Geometry check sheet. Reference: the model listing, model coordinates, mm. A direction names the side the tool comes from. Give positions to 0.01 mm unless a question says otherwise; leave off trailing zeros. Write each loop counter-clockwise with the first axis right and the second up, starting at its lowest first coordinate (ties: lowest second). Pieces come first, ordered by that corner, then holes. Notation, with made-up numbers: (-21.75, -16) - (34.25, -16) arc R25 ccw to (34.25, 18) - close; hole circle Ø4 at (32, 18.5). An arc over 180 degrees is marked (long way). One line per question, with ' | ' between items. Start each with the question number.
Q1. Set-up check for faces 1 (the face through (5.309, -99, 26)), 2 (the face through (71.725, -198.341, 2.691)), 3 (the face through (58, -183.388, 3)): record each of +Z, -Z, +X, -X, +Y, -Y from which the full face is reachable in a straight line by a thin tool's end or side.
Q2. Release check for a two-part mould opening along X. For faces 4 (the face through (58, -30.988, 3)), 5 (the face through (2.62, -1.81, 41.5)), 6 (the face through (0, -99, 23)) record: +X half, -X half, draft (parallel to the pull), parting line (faces both ways), or undercut.
Q3. Section check C-C on z = 32.5. Record the boundary of the cut face in (x, y).
Q4. Section check D-D on y = -179.5. Record the boundary of the cut face in (x, z).
Q5. Gauge pin test, flat ends, axial feed: P1, Ø19.5, axis at x = 45, y = -150, coming from the +Z side; P2, Ø5, axis at x = 35.5, z = 7, coming from the +Y side; P3, Ø13, axis at y = -74.68, z = 29.92, coming from the -X side. Record the tip position at first contact, or that the pin passes through.
Q6. Section check A-A on y = -73.5. Record the boundary of the cut face in (x, z), and give its area (3 significant figures).
Q7. Thickness scan on L1, parallel to Y at x = 53, z = 3.5; L2, parallel to Z at x = 22, y = -143.5. Record the ranges inside material, lowest first. Write a range as [from, to].
Q8. Section check B-B on y = -140. Record the boundary of the cut face in (x, z), and give its area (3 significant figures).
```python
from build123d import *

# Parameters (mm, degrees)
F1_DEPTH = 200.152
F3_D     = 14.3002
F4_R     = 6.35
F6_DEPTH = 25.4


with BuildPart() as f1:
    # F0 (on Front) → F1 (new body)
    with BuildSketch(Plane.XZ):
        with BuildLine():
            ThreePointArc((0, 2.794), (0.818344, 0.818344), (2.794, 0))
            Line((2.794, 0), (73.6346, 0))
            Line((73.6346, 0), (73.6346, 5.3086))
            Line((73.6346, 5.3086), (8.1026, 5.3086))
            ThreePointArc((8.1026, 5.3086), (6.126944, 6.126944), (5.3086, 8.1026))
            Line((5.3086, 8.1026), (5.3086, 43.4086))
            Line((5.3086, 43.4086), (0, 43.4086))
            Line((0, 43.4086), (0, 2.794))
        make_face()
    extrude(amount=F1_DEPTH)

    # F3 (through all)
    with Locations(Plane(origin=(0, 0, 0), x_dir=(0, -1, 0), z_dir=(-1, 0, 0))):
        with Locations((23.876, 29.9212), (74.676, 29.9212), (125.476, 29.9212), (176.276, 29.9212)):
            Hole(F3_D / 2)

    # F4
    f4_edges = [f1.edges().sort_by_distance(p)[0] for p in [
        (2.6543, 0, 43.4086),
        (73.6346, 0, 2.6543),
        (73.6346, -200.152, 2.6543),
        (2.6543, -200.152, 43.4086),
    ]]
    fillet(f4_edges, radius=F4_R)

    # F5 (on face) → F6 (cut)
    with BuildSketch(Plane.XY.offset(5.3086)):
        with BuildLine():
            ThreePointArc((66.3956, -23.876), (64.312543, -18.847057), (59.2836, -16.764))
            Line((59.2836, -16.764), (55.9816, -16.764))
            ThreePointArc((55.9816, -16.764), (50.952657, -18.847057), (48.8696, -23.876))
            ThreePointArc((48.8696, -23.876), (50.952657, -28.904943), (55.9816, -30.988))
            Line((55.9816, -30.988), (59.2836, -30.988))
            ThreePointArc((59.2836, -30.988), (64.312543, -28.904943), (66.3956, -23.876))
        make_face()
        with BuildLine():
            ThreePointArc((66.3956, -176.276), (64.312543, -171.247057), (59.2836, -169.164))
            Line((59.2836, -169.164), (55.9816, -169.164))
            ThreePointArc((55.9816, -169.164), (50.952657, -171.247057), (48.8696, -176.276))
            ThreePointArc((48.8696, -176.276), (50.952657, -181.304943), (55.9816, -183.388))
            Line((55.9816, -183.388), (59.2836, -183.388))
            ThreePointArc((59.2836, -183.388), (64.312543, -181.304943), (66.3956, -176.276))
        make_face()
    extrude(amount=-F6_DEPTH, mode=Mode.SUBTRACT)


solid = f1.part
```
Working result:
1) face 1: +Z, +X, +Y, -Y | face 2: +Z, -Z, +X, -Y | face 3: +Z, -Z
2) face 4: undercut | face 5: draft | face 6: -X half
3) outline: (0, -200.15) - (5.31, -200.15) - (5.31, -182.94) - (0, -182.94) - close; (0, -169.61) - (5.31, -169.61) - (5.31, -132.14) - (0, -132.14) - close; (0, -118.81) - (5.31, -118.81) - (5.31, -81.34) - (0, -81.34) - close; (0, -68.01) - (5.31, -68.01) - (5.31, -30.54) - (0, -30.54) - close; (0, -17.21) - (5.31, -17.21) - (5.31, 0) - (0, 0) - close
4) outline: (0, 2.79) arc R2.79 ccw to (2.79, 0) - (49.64, 0) - (49.64, 5.31) - (8.1, 5.31) arc R2.79 cw to (5.31, 8.1) - (5.31, 23.54) - (0, 23.54) - close; (0, 36.3) - (5.31, 36.3) - (5.31, 43.41) - (0, 43.41) - close; (65.62, 0) - (73.63, 0) - (73.63, 5.31) - (65.62, 5.31) - close
5) P1: stops at z = 5.31 | P2: stops at y = 0 | P3: passes through
6) outline: (0, 2.79) arc R2.79 ccw to (2.79, 0) - (73.63, 0) - (73.63, 5.31) - (8.1, 5.31) arc R2.79 cw to (5.31, 8.1) - (5.31, 22.87) - (0, 22.87) - close; (0, 36.97) - (5.31, 36.97) - (5.31, 43.41) - (0, 43.41) - close | area: 518 mm2
7) L1: y = [-200.15, -182.73], [-169.82, -30.33], [-17.42, 0] | L2: z = [0, 5.31]
8) outline: (0, 2.79) arc R2.79 ccw to (2.79, 0) - (73.63, 0) - (73.63, 5.31) - (8.1, 5.31) arc R2.79 cw to (5.31, 8.1) - (5.31, 43.41) - (0, 43.41) - close | area: 593 mm2
